For this review, use the dimensioned drawing (mm, ordinates from the lowest corner) and the shaded views. Coordinates: 2 decimals unless noted, no trailing zeros. Order: outer loops, then holes, each group sorted by start corner. A loop starts at its lowest first (then second) coordinate and runs counter-clockwise, first axis right, second up. Notation, with made-up numbers: (-5, -0.75) -> (43, -0.75) arc R15 ccw to (43, 10.25) -> close; hole circle Ø1 at (29, 35.5). An arc over 180 degrees is marked (long way). Use one line per item in the form item = value. Start each with the question number.
(1) Wall thickness on line 1 along X through (y, z) = (28.5, 98): over which ranges is the line inside the solid? List them lowest first.
(2) Insertion check: pin 1 Ø25 at (y, z) = (21, 40) entering from +X; pin 2 Ø15 at (y, z) = (28.5, 51.5) entering from -X. Each pin has a flat end and moves straight along its axis. Give the tip position at first contact, or say it passes through.
(3) Take a section at C-C (y = 30). State the section outline as (x, z) points.
(4) Take a section at D-D (z = 75). State the section outline as (x, y) points, then the cut area to 3 significant figures.
(5) Take a section at A-A (z = 25). State the section outline as (x, y) points, then the cut area to 3 significant figures.
(6) Take a section at B-B (x = 8). State the section outline as (y, z) points.
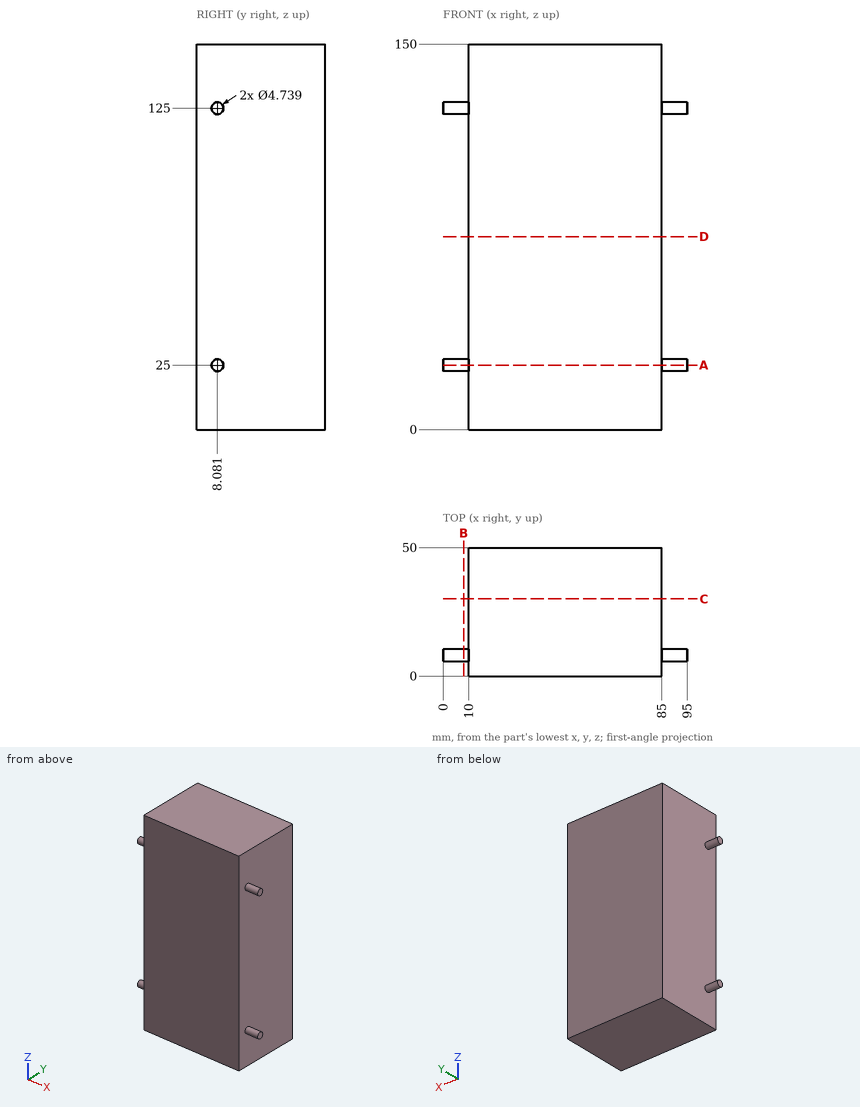
Findings:
q1.line_1 = 10 to 85
q2.pin_1 = 85
q2.pin_2 = 10
q3.outline = (10, 0) -> (85, 0) -> (85, 150) -> (10, 150) -> close
q4.outline = (10, 0) -> (85, 0) -> (85, 50) -> (10, 50) -> close
q4.area = 3,750 mm²
q5.outline = (0, 5.71) -> (10, 5.71) -> (10, 0) -> (85, 0) -> (85, 5.71) -> (95, 5.71) -> (95, 10.45) -> (85, 10.45) -> (85, 50) -> (10, 50) -> (10, 10.45) -> (0, 10.45) -> close
q5.area = 3,840 mm²
q6.outline = circle Ø4.74 at (8.08, 25); circle Ø4.74 at (8.08, 125)
